Study the drawing (mm; zero at the part's minimum x, y, z) and answer. Round coordinates to 2 decimals unless told otherwise and drop trailing zeros. Order: outer loops, then holes, each group sorted by start corner. A loop starts at its lowest first (then second) coordinate and runs counter-clockwise, first axis right, second up. Notation, with made-up numbers: (87, 60) - (122, 60) arc R34 ccw to (122, 93) - close; hole circle Ø11 at (-5.75, -2.5). An arc over 180 degrees is marked (long way). Put each result on its own line as item: value.
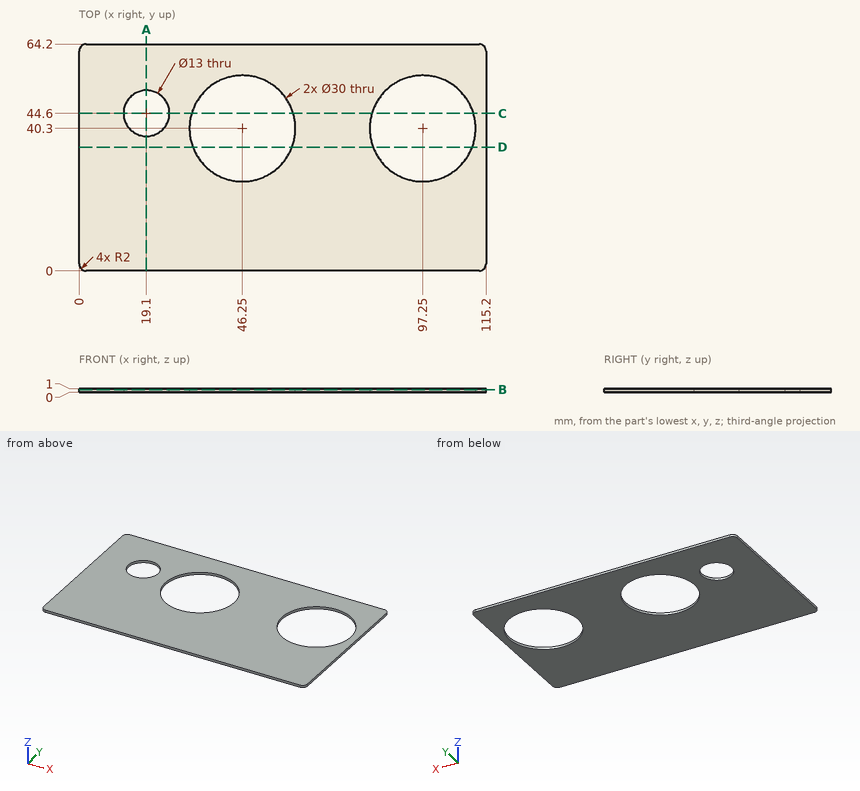
1) Given pin 1 Ø1 at (x, y) = (78, 30.5) entering from -Z; pin 2 Ø4 at (x, y) = (56.5, 34.5) entering from +Z, each flat-ended and moving along its own axis, determine where each tip first touches the part or whether it passes through.
Findings below:
pin 1: stops at z = 0
pin 2: passes through
2) A cutting plane is placed at B-B on z = 0.8. Write down the section's boundary in (x, y), then the cut area to 3 significant figures.
Findings below:
outline: (0, 2) arc R2 ccw to (2, 0) - (113.2, 0) arc R2 ccw to (115.2, 2) - (115.2, 62.2) arc R2 ccw to (113.2, 64.2) - (2, 64.2) arc R2 ccw to (0, 62.2) - close; hole circle Ø13 at (19.1, 44.6); hole circle Ø30 at (46.25, 40.3); hole circle Ø30 at (97.25, 40.3)
area: 5,850 mm2
3) Straight lines are drawn through the part: L1, parallel to X at y = 32.5, z = 0.9; L2, parallel to X at y = 32, z = 0.9; L3, parallel to X at y = 41, z = 0.75. For each, find the intervals that lie inside material, in ascending order. Write a range as from..to.
Findings below:
L1: x = 0..33.44, 59.06..84.44, 110.06..115.2
L2: x = 0..33.76, 58.74..84.76, 109.74..115.2
L3: x = 0..13.69, 24.51..31.27, 61.23..82.27, 112.23..115.2
4) A cutting plane is placed at D-D on y = 35. Write down the section's boundary in (x, z), then the cut area to 3 significant figures.
Findings below:
outline: (0, 0) - (32.22, 0) - (32.22, 1) - (0, 1) - close; (60.28, 0) - (83.22, 0) - (83.22, 1) - (60.28, 1) - close; (111.28, 0) - (115.2, 0) - (115.2, 1) - (111.28, 1) - close
area: 59.1 mm2
5) A cutting plane is placed at A-A on x = 19.1. Write down the section's boundary in (y, z), then the cut area to 3 significant figures.
Findings below:
outline: (0, 0) - (38.1, 0) - (38.1, 1) - (0, 1) - close; (51.1, 0) - (64.2, 0) - (64.2, 1) - (51.1, 1) - close
area: 51.2 mm2
6) A cutting plane is placed at C-C on y = 44.6. Write down the section's boundary in (x, z), then the cut area to 3 significant figures.
Findings below:
outline: (0, 0) - (12.6, 0) - (12.6, 1) - (0, 1) - close; (25.6, 0) - (31.88, 0) - (31.88, 1) - (25.6, 1) - close; (60.62, 0) - (82.88, 0) - (82.88, 1) - (60.62, 1) - close; (111.62, 0) - (115.2, 0) - (115.2, 1) - (111.62, 1) - close
area: 44.7 mm2
